Autodesk Inventor part; units mm, degrees
ref_plane "YZ Plane" through (0, 0, 0) normal (1, 0, 0) x (0, 1, 0)
ref_plane "XZ Plane" through (0, 0, 0) normal (0, 1, 0) x (-1, 0, 0)
ref_plane "XY Plane" through (0, 0, 0) normal (0, 0, 1) x (1, 0, 0)
sketch "Sketch1" plane through (0, 0, 0) normal (0, 1, 0) x (-1, 0, 0)
  line L0 (0, 0) -> (-100, 0)
  line L1 (-100, 0) -> (-100, 50)
  line L2 (-100, 50) -> (0, 50)
  line L3 (0, 50) -> (0, 0)
  dimension "d0" = 100
  dimension "d1" = 50
extrude "Extrusion1" add sketch "Sketch1" along normal blind 5
sketch "Sketch3" plane through (0, 5, 0) normal (0, 1, 0) x (1, 0, 0)
  line L0 (0, -50) -> (100, -50)
  line L1 (0, 0) -> (5, 0)
  line L2 (5, 0) -> (5, -50)
  line L3 (5, -50) -> (0, -50)
  line L4 (0, -50) -> (0, 0)
  dimension "d14" = 5
extrude "Extrusion2" add sketch "Sketch3" along normal blind 50
sketch "Sketch4" plane through (0, 5, 0) normal (0, 1, 0) x (1, 0, 0)
  line L0 (5, 0) -> (5, -50)
  line L1 (5, -50) -> (100, -50) construction
  line L2 (100, -50) -> (100, 0) construction
  line L3 (100, 0) -> (5, 0) construction
  arc A0 (78.411, -28) -> (78.411, -22) centre (78.411, -25) ccw
  arc A1 (22.5222, -22) -> (22.5222, -28) centre (22.5222, -25) ccw
  line L4 (22.5222, -22) -> (78.411, -22)
  line L5 (78.411, -28) -> (22.5222, -28)
  point P0 (0, 0)
  point P1 (100, -25)
  dimension "d30" = 6
  dimension "d31" = 6
  dimension "d32" = 25
extrude "Extrusion3" cut sketch "Sketch4" against normal up to surface (5 mm away)
properties part number "Horonyrogzito_b"
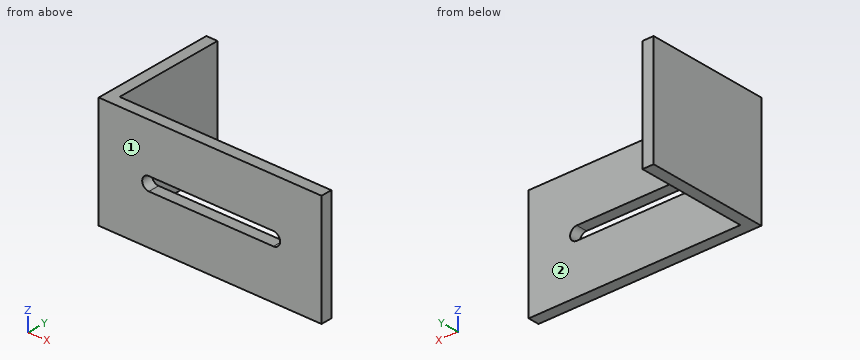
Part model, mm, in its own coordinate system. Face numbers are marked on the shaded views. A direction names the side the tool comes from. Round coordinates to 2 decimals unless told otherwise and drop trailing zeros. Loops run counter-clockwise (first coordinate to the right, second up) from the corner with the lowest first, then second, coordinate; pieces in that order, holes last.
1. Slice it at A-A (z = 25). Give the cut face in (x, y), and give its area (3 significant figures).
Solutions:
outline: (0, 0) - (19.52, 0) - (19.52, 5) - (5, 5) - (5, 55) - (0, 55) - close; (81.41, 0) - (100, 0) - (100, 5) - (81.41, 5) - close
area: 441 mm2
2. 3-axis set-ups, long thin cutter, end or side, ignore diameter. For the marked faces 1 and 2: which of +Z, -Z, +X, -X, +Y, -Y reach the whole face in a straight line?
Solutions:
face 1: +Z, -Z, +X, -X, -Y
face 2: +Z, -Z, +X, +Y
3. Slice it at D-D (z = 6.5). Give the cut face in (x, y).
Solutions:
outline: (0, 0) - (100, 0) - (100, 5) - (5, 5) - (5, 55) - (0, 55) - close
4. Slice it at B-B (x = 77). Give the cut face in (y, z).
Solutions:
outline: (0, 0) - (5, 0) - (5, 22) - (0, 22) - close; (0, 28) - (5, 28) - (5, 50) - (0, 50) - close
5. Flat gauge pins, fed straight in: pin 1 (3 mm diameter, centred on y = 28.5, z = 12, fed in from +X); pin 2 (2.5 mm diameter, centred on x = 48, y = 3.5, fed in from -Z); pin 3 (10 mm diameter, centred on x = 77, z = 39.5, fed in from +Y). Where does each tip first touch, or does it go through?
Solutions:
pin 1: stops at x = 5
pin 2: stops at z = 0
pin 3: stops at y = 5
6. Drill centre line: line 1 along Y through (x, z) = (70.5, 41.5). Where is it in solid material? Low to high.
Solutions:
line 1: y = 0 to 5
7. Slice it at C-C (x = 15). Give the cut face in (y, z).
Solutions:
outline: (0, 0) - (5, 0) - (5, 50) - (0, 50) - close
